```python
from build123d import *

# Parameters (mm, degrees)
SKETCH1_R           = 60.5
BOSS_EXTRUDE1_DEPTH = 19
SKETCH2_R           = 0.5
CUT_EXTRUDE2_DEPTH  = 20


with BuildPart() as part:
    # Sketch1 → Boss-Extrude1 (new body)
    with BuildSketch(Plane(origin=(0, 0, 0), x_dir=(1, 0, 0), z_dir=(0, 1, 0))):
        Circle(SKETCH1_R)
    extrude(amount=BOSS_EXTRUDE1_DEPTH)

    # Sketch2 → Cut-Extrude2 (cut, through all)
    with BuildSketch(Plane(origin=(0, 19, 0), x_dir=(1, 0, 0), z_dir=(0, 1, 0))):
        with Locations((-8.660254038, 5)):
            Circle(SKETCH2_R)
        with Locations((8.660254038, 5)):
            Circle(SKETCH2_R)
        with Locations((0, -10)):
            Circle(SKETCH2_R)
        Polygon((0, 7.2), (6.235382907, -3.6), (-6.235382907, -3.6), align=None)
    extrude(amount=-CUT_EXTRUDE2_DEPTH, mode=Mode.SUBTRACT)


solid = part.part
```
Here's how the part is built. I have some questions about the finished solid (model axes, mm). A direction names the side the tool comes from. Coordinates: 2 decimals unless noted, no trailing zeros. Order: outer loops, then holes, each group sorted by start corner. A loop starts at its lowest first (then second) coordinate and runs counter-clockwise, first axis right, second up.
Item 1: I'm going to push flat-ended pins straight in: pin 1 Ø8 at (x, y) = (-16, 8.5) entering from +Z; pin 2 Ø1 at (y, z) = (3, -24) entering from -X; pin 3 Ø3 at (x, y) = (-3.5, 15.5) entering from +Z. Where does each tip first touch, or does it pass through?
Response values:
pin 1: stops at z = 59.3
pin 2: stops at x = -55.75
pin 3: stops at z = 60.47
Item 2: If we section it at D-D, the plane z = 16: List the corners of the cut face in (x, y) for me, then the cut area to 3 significant figures.
Response values:
outline: (-58.35, 0) - (58.35, 0) - (58.35, 19) - (-58.35, 19) - close
area: 2,220 mm2
Item 3: If we section it at A-A, the plane y = 7.5: List the corners of the cut face in (x, z) for me, then the cut area to 3 significant figures.
Response values:
outline: circle Ø121 at (0, 0); hole circle Ø1 at (-8.66, -5); hole (-6.24, 3.6) - (0, -7.2) - (6.24, 3.6) - close; hole circle Ø1 at (0, 10); hole circle Ø1 at (8.66, -5)
area: 11,400 mm2
Item 4: If we section it at C-C, the plane x = -18.5: List the corners of the cut face in (y, z) for me, then the cut area to 3 significant figures.
Response values:
outline: (0, -57.6) - (19, -57.6) - (19, 57.6) - (0, 57.6) - close
area: 2,190 mm2
Item 5: Which directions (+Z, -Z, +X, -X, +Y, -Y) give clear straight access to the entire face, cutting with the end or side of a thin tool? Please do faces 1 (the face through (13, 0, -1)), 2 (the face through (0, 10, 3.6)).
Response values:
face 1: +Z, -Z, +X, -X, -Y
face 2: +Y, -Y
Item 6: I need wall thicknesses on probe 1 along Z at (x, y) = (0, 5); probe 2 along X at (y, z) = (9.5, -5); probe 3 along Z at (x, y) = (-3, 13.25). Which ranges of each line are inside material? Lowest first, please.
Response values:
probe 1: z = -60.5 to -7.2, 3.6 to 9.5, 10.5 to 60.5
probe 2: x = -60.29 to -9.16, -8.16 to -1.27, 1.27 to 8.16, 9.16 to 60.29
probe 3: z = -60.43 to -2, 3.6 to 60.43
Item 7: If we section it at B-B, the plane z = 0: List the corners of the cut face in (x, y) for me.
Response values:
outline: (-60.5, 0) - (-4.16, 0) - (-4.16, 19) - (-60.5, 19) - close; (4.16, 0) - (60.5, 0) - (60.5, 19) - (4.16, 19) - close
Item 8: Thinking about a two-plate mould opening in X: for faces 3 (the face through (-3, 10, -2)), 4 (the face through (13, 19, -1)), 5 (the face through (-13.12, 9.37, 59.06)), which applies, pulls with the +X half, pulls with the -X half, needs draft (parallel to the pull), parting line crosses it, or undercut?
Response values:
face 3: undercut
face 4: needs draft
face 5: parting line crosses it
